The listing builds one solid part. Answer for the finished solid, in the listing's coordinates (mm). Face numbers are marked on the shaded views. A direction names the side the tool comes from. Round coordinates to 2 decimals unless told otherwise and drop trailing zeros. Order: outer loops, then holes, each group sorted by start corner. A loop starts at its lowest first (then second) coordinate and runs counter-clockwise, first axis right, second up. Notation, with made-up numbers: M 68.5,-26.75 L 95.5,-26.75 A22 cw 95.5,2.25 Z; hole C -14.5,-32 d9. An arc over 180 degrees is marked long. Put each result on its own line as item: value. Start each with the question number.
1. The part is cut by section D-D (x = -8.25). Give the vertices of the cut face in (y, z), then the cut area to 3 significant figures.
2. Which of the six approach directions +Z, -Z, +X, -X, +Y, -Y give full straight-line access (tool end or side, diameter ignored) to the marked faces 5 and 6?
3. The part is cut by section B-B (z = -0.95). Give the vertices of the cut face in (x, y).
4. Consider line 1 (Y direction, x = 0, z = 0.45); line 2 (X direction, y = 0, z = 0.55); line 3 (Z direction, x = -7.5, y = 4). Determine where each line is inside the solid, lowest interval first.
5. The part is cut by section C-C (y = 4.5). Give the vertices of the cut face in (x, z).
6. This flat-tipped pin is pushed along its axis until it touches: pin 1 Ø5.5 at (x, y) = (0, 0) entering from -Z. Where does it stop, or does it pass through?
7. The mould has two halves that part along X. Classify the marked faces 1, 2, 3 and 4: +X half, -X half, draft (parallel to the pull), parting line (faces both ways), or undercut.
8. The part is cut by section A-A (x = 0). Give the vertices of the cut face in (y, z) (3 decimals), then the cut area to 3 significant figures.
from build123d import *

# Parameters (mm, degrees)
BOSS_EXTRUDE1_DEPTH      = 1.1938
BOSS_EXTRUDE1_DEPTH_BACK = 1.1938
SKETCH2_R                = 3.5687
BOSS_EXTRUDE2_DEPTH      = 1.9558


with BuildPart() as part:
    # Sketch1 → Boss-Extrude1 (new body, two sides)
    with BuildSketch(Plane.XY) as boss_extrude1_sk:
        with BuildLine():
            Line((-7.0739, -5.6261), (7.0739, -5.6261))
            ThreePointArc((7.0739, -5.6261), (12.7, 0), (7.0739, 5.6261))
            Line((7.0739, 5.6261), (-7.0739, 5.6261))
            ThreePointArc((-7.0739, 5.6261), (-12.7, 0), (-7.0739, -5.6261))
        make_face()
    extrude(amount=BOSS_EXTRUDE1_DEPTH)
    extrude(boss_extrude1_sk.sketch, amount=-BOSS_EXTRUDE1_DEPTH_BACK)

    # Sketch2 → Boss-Extrude2 (add)
    with BuildSketch(Plane.XY):
        Circle(SKETCH2_R)
    extrude(amount=BOSS_EXTRUDE2_DEPTH)

    # Sketch3 → Cut-Revolve1 (revolve, cut)
    with BuildSketch(Plane(origin=(0, 0, 0), x_dir=(0, 0, -1), z_dir=(1, 0, 0))):
        Polygon((-1.9558, 0), (-1.9558, 3.175), (-1.26873, 2.48793), (0.50673, 2.48793), (1.1938, 3.175), (1.1938, 0), align=None)
    revolve(axis=Axis((0, 0, -1.1938), (0, 0, 1)), mode=Mode.SUBTRACT)


solid = part.part
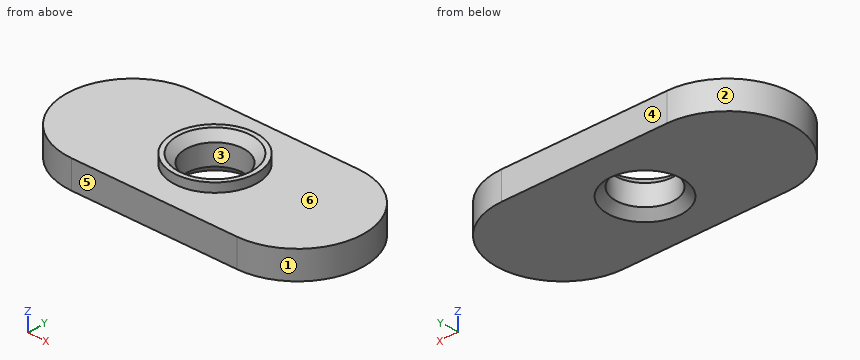
Resolved:
1. outline: M -5.5,-1.19 L 5.5,-1.19 L 5.5,1.19 L -5.5,1.19 Z
1. area: 26.3 mm2
2. face 5: +Z, -Z, +X, -X, -Y
2. face 6: +Z
3. outline: M -7.07,-5.63 L 7.07,-5.63 A5.63 ccw 7.07,5.63 L -7.07,5.63 A5.63 ccw Z; hole C 0,0 d5.86
4. line 1: -5.63 to -2.49, 2.49 to 5.63
4. line 2: -12.7 to -2.49, 2.49 to 12.7
4. line 3: -1.19 to 1.19
5. outline: M -10.45,-1.19 L 10.45,-1.19 L 10.45,1.19 L -10.45,1.19 Z
6. pin 1: z = -0.77
7. face 1: +X half
7. face 2: -X half
7. face 3: undercut
7. face 4: draft
8. outline: M -5.626,-1.194 L -3.175,-1.194 L -2.488,-0.507 L -2.488,1.269 L -3.175,1.956 L -3.569,1.956 L -3.569,1.194 L -5.626,1.194 Z; M 2.488,-0.507 L 3.175,-1.194 L 5.626,-1.194 L 5.626,1.194 L 3.569,1.194 L 3.569,1.956 L 3.175,1.956 L 2.488,1.269 Z
8. area: 15.7 mm2
